from build123d import *

# Parameters (mm, degrees)
SKETCH_1_W          = 110
SKETCH_1_H          = 25
SKETCH_1_R          = 1.6
EXTRUDE_1_DEPTH     = 2
SKETCH_2_W          = 60
SKETCH_2_H          = 15
EXTRUDE_2_DEPTH     = 113
CUT_EXTRUDE_1_DEPTH = 60
FILLET_1_R          = 2
FILLET_2_R          = 2
FILLET_3_R          = 2
FILLET_4_R          = 2


with BuildPart() as part:
    # 草图1 → 凸台-拉伸1 (new body)
    with BuildSketch(Plane(origin=(0, 0, 0), x_dir=(1, 0, 0), z_dir=(0, 1, 0))):
        Rectangle(SKETCH_1_W, SKETCH_1_H)
        with Locations(Location((-49, 7.5, 0), (0, 0, 270))):
            Circle(SKETCH_1_R, mode=Mode.SUBTRACT)
        with Locations(Location((49, 7.5, 0), (0, 0, 90))):
            Circle(SKETCH_1_R, mode=Mode.SUBTRACT)
        with Locations(Location((49, -7.5, 0), (0, 0, 270))):
            Circle(SKETCH_1_R, mode=Mode.SUBTRACT)
        with Locations(Location((-49, -7.5, 0), (0, 0, 90))):
            Circle(SKETCH_1_R, mode=Mode.SUBTRACT)
    extrude(amount=EXTRUDE_1_DEPTH)

    # 草图2 → 凸台-拉伸2 (add)
    with BuildSketch(Plane(origin=(0, 115, 0), x_dir=(1, 0, 0), z_dir=(0, 1, 0))):
        with Locations((0, 5)):
            Rectangle(SKETCH_2_W, SKETCH_2_H)
    extrude(amount=-EXTRUDE_2_DEPTH)

    # 草图3 → 切除-拉伸1 (cut)
    with BuildSketch(Plane(origin=(30, 0, 0), x_dir=(0, 0, -1), z_dir=(1, 0, 0))):
        Polygon((-2.5, 36), (-1.5, 36), (-1.5, 34), (10.1, 34), (10.1, 113), (-1.5, 113), (-1.5, 111), (-2.5, 111), align=None)
    extrude(amount=-CUT_EXTRUDE_1_DEPTH, mode=Mode.SUBTRACT)

    # 圆角1
    fillet_1_edges = [part.edges().sort_by_distance(p)[0] for p in [
        (55, 1, 12.5),
    ]]
    fillet(fillet_1_edges, radius=FILLET_1_R)

    # 圆角2
    fillet_2_edges = [part.edges().sort_by_distance(p)[0] for p in [
        (55, 1, -12.5),
    ]]
    fillet(fillet_2_edges, radius=FILLET_2_R)

    # 圆角3
    fillet_3_edges = [part.edges().sort_by_distance(p)[0] for p in [
        (-55, 1, -12.5),
    ]]
    fillet(fillet_3_edges, radius=FILLET_3_R)

    # 圆角4
    fillet_4_edges = [part.edges().sort_by_distance(p)[0] for p in [
        (-55, 1, 12.5),
    ]]
    fillet(fillet_4_edges, radius=FILLET_4_R)


solid = part.part
Verification items for the finished model (mm, model axes). A direction names the side the tool comes from. Coordinates: 2 decimals unless noted, no trailing zeros. Order: outer loops, then holes, each group sorted by start corner. A loop starts at its lowest first (then second) coordinate and runs counter-clockwise, first axis right, second up.
1. Sectioned sample at B-B, the plane z = -7.5. Record the cut outline in (x, y).
Results found:
outline: (-55, 0) - (-50.6, 0) - (-50.6, 2) - (-55, 2) - close; (-47.4, 0) - (47.4, 0) - (47.4, 2) - (30, 2) - (30, 34) - (-30, 34) - (-30, 2) - (-47.4, 2) - close; (-30, 113) - (30, 113) - (30, 115) - (-30, 115) - close; (50.6, 0) - (55, 0) - (55, 2) - (50.6, 2) - close
2. Sectioned sample at D-D, the plane x = -24. Record the cut outline in (y, z), and give its area (3 significant figures).
Results found:
outline: (0, -12.5) - (115, -12.5) - (115, 2.5) - (111, 2.5) - (111, 1.5) - (113, 1.5) - (113, -10.1) - (34, -10.1) - (34, 1.5) - (36, 1.5) - (36, 2.5) - (2, 2.5) - (2, 12.5) - (0, 12.5) - close
area: 754 mm2
3. Release check for a two-part mould opening along Z. For faces 6 (the face through (-1, 0, 0)), 7 (the face through (0, 113, -4)), 8 (the face through (0, 113, 2.5)) record: +Z half, -Z half, draft (parallel to the pull), parting line (faces both ways), or undercut.
Results found:
face 6: draft
face 7: undercut
face 8: +Z half
4. Scan lines: line 1 (X direction, y = 0.9, z = -7.5); line 2 (Y direction, x = -5, z = -0.5); line 3 (Z direction, x = -25, y = 65). Record each from-to range of solid material in increasing order.
Results found:
line 1: x = -55 to -50.6, -47.4 to 47.4, 50.6 to 55
line 2: y = 0 to 34, 113 to 115
line 3: z = -12.5 to -10.1
5. Sectioned sample at A-A, the plane x = 49. Record the cut outline in (y, z).
Results found:
outline: (0, -12.5) - (2, -12.5) - (2, -9.1) - (0, -9.1) - close; (0, -5.9) - (2, -5.9) - (2, 5.9) - (0, 5.9) - close; (0, 9.1) - (2, 9.1) - (2, 12.5) - (0, 12.5) - close
6. Set-up check for faces 1 (the face through (-30, 38, -11)), 2 (the face through (0, 19, 2.5)), 3 (the face through (30, 38, -11)), 4 (the face through (0, 34, -4)), 5 (the face through (0, 115, -5)): record each of +Z, -Z, +X, -X, +Y, -Y from which the full face is reachable in a straight line by a thin tool's end or side.
Results found:
face 1: +Z, -Z, -X, +Y
face 2: +Z, +X, -X, +Y
face 3: +Z, -Z, +X, +Y
face 4: +X, -X
face 5: +Z, -Z, +X, -X, +Y
7. Go/stop test with flat-tipped pins: pin 1 Ø10 at (y, z) = (45.5, -5.5) entering from -X; pin 2 Ø2 at (x, y) = (-8.5, 114) entering from +Z; pin 3 Ø10 at (x, z) = (38, 6.5) entering from +Y. Record where each tip stops, or that it passes through.
Results found:
pin 1: stops at x = -30
pin 2: stops at z = 2.5
pin 3: stops at y = 2
8. Sectioned sample at C-C, the plane z = 7.5. Record the cut outline in (x, y), and give its area (3 significant figures).
Results found:
outline: (-55, 0) - (-50.6, 0) - (-50.6, 2) - (-55, 2) - close; (-47.4, 0) - (47.4, 0) - (47.4, 2) - (-47.4, 2) - close; (50.6, 0) - (55, 0) - (55, 2) - (50.6, 2) - close
area: 207 mm2
